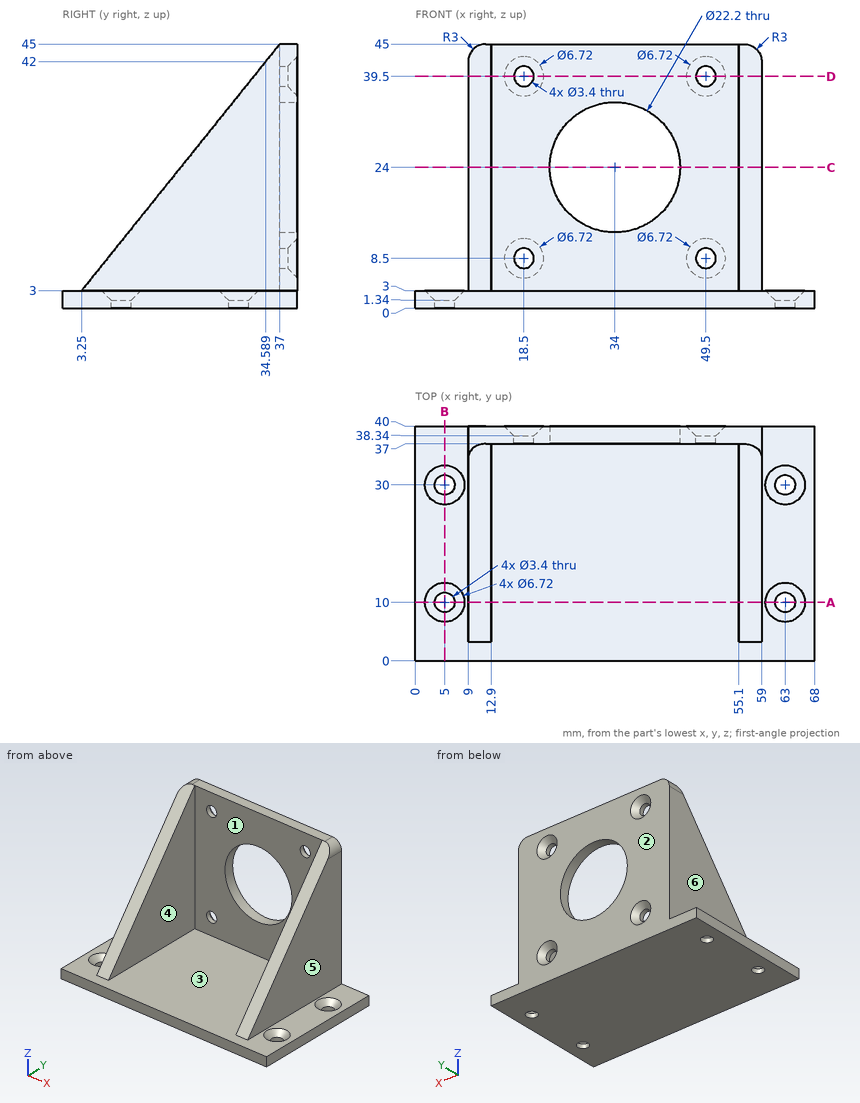
Geometry: see drawing. Coordinates: mm, zero at the bounding-box minimum. A direction names the side the tool comes from. Round coordinates to 2 decimals unless told otherwise and drop trailing zeros. Write each loop counter-clockwise with the first axis right and the second up, starting at its lowest first coordinate (ties: lowest second). Pieces come first, ordered by that corner, then holes.
1) Draft query along Y for the marked faces 1, 2 and 3. Return one class per face: pulls with the +Y half, pulls with the -Y half, needs draft (parallel to the pull), parting line crosses it, or undercut.
2) Cut plane D-D (z = 39.5). Return the cut outline in (x, y).
3) Reachability of the marked faces 4, 5 and 6 from +Z, -Z, +X, -X, +Y, -Y: full face, straight path, thin tool, end or side. Return the list, or none.
4) Cut plane B-B (x = 5). Return the cut outline in (y, z).
5) Ray query, L1, parallel to X at y = 37.6, z = 39.5; L2, parallel to X at y = 10, z = 0.8; L3, parallel to Z at x = 18.5, y = 37.8. Return the intervals inside material, ascending.
6) Contact query for flat-ended pins moving along their axis: P1, Ø5.5, axis at x = 49.5, z = 39.5, coming from the +Y side; P2, Ø3, axis at x = 63, y = 10, coming from the -Z side; P3, Ø4, axis at x = 63, y = 30, coming from the +Z side; P4, Ø2, axis at x = 22, z = 7, coming from the -Y side. Output: stop coordinate, or through.
7) Cut plane C-C (z = 24). Return the cut outline in (x, y) (1 decimal).
8) Cut plane A-A (y = 10). Return the cut outline in (x, z), then the cut area to 3 significant figures.
Geometry says:
1. face 1: pulls with the -Y half
1. face 2: pulls with the +Y half
1. face 3: needs draft
2. outline: (9, 32.58) - (12.9, 32.58) - (12.9, 37) - (16.8, 37) - (16.8, 38.34) - (15.14, 40) - (9, 40) - close; (20.2, 37) - (47.8, 37) - (47.8, 38.34) - (46.14, 40) - (21.86, 40) - (20.2, 38.34) - close; (51.2, 37) - (55.1, 37) - (55.1, 32.58) - (59, 32.58) - (59, 40) - (52.86, 40) - (51.2, 38.34) - close
3. face 4: +Z, -Y
3. face 5: +Z, +X, +Y, -Y
3. face 6: +Z, -X, +Y, -Y
4. outline: (0, 0) - (8.3, 0) - (8.3, 1.34) - (6.64, 3) - (0, 3) - close; (11.7, 0) - (28.3, 0) - (28.3, 1.34) - (26.64, 3) - (13.36, 3) - (11.7, 1.34) - close; (31.7, 0) - (40, 0) - (40, 3) - (33.36, 3) - (31.7, 1.34) - close
5. L1: x = 9 to 16.8, 20.2 to 47.8, 51.2 to 59
5. L2: x = 0 to 3.3, 6.7 to 61.3, 64.7 to 68
5. L3: z = 0 to 6.8, 10.2 to 37.8, 41.2 to 45
6. P1: stops at y = 39.39
6. P2: passes through
6. P3: stops at z = 1.64
6. P4: stops at y = 37
7. outline: (9, 20.1) - (12.9, 20.1) - (12.9, 37) - (22.9, 37) - (22.9, 40) - (9, 40) - close; (45.1, 37) - (55.1, 37) - (55.1, 20.1) - (59, 20.1) - (59, 40) - (45.1, 40) - close
8. outline: (0, 0) - (3.3, 0) - (3.3, 1.34) - (1.64, 3) - (0, 3) - close; (6.7, 0) - (61.3, 0) - (61.3, 1.34) - (59.64, 3) - (59, 3) - (59, 11.4) - (55.1, 11.4) - (55.1, 3) - (12.9, 3) - (12.9, 11.4) - (9, 11.4) - (9, 3) - (8.36, 3) - (6.7, 1.34) - close; (64.7, 0) - (68, 0) - (68, 3) - (66.36, 3) - (64.7, 1.34) - close
8. area: 244 mm2
